Here's how the part is built. I have some questions about the finished solid (model axes, mm). A direction names the side the tool comes from. Round coordinates to 2 decimals unless told otherwise and drop trailing zeros. Order: outer loops, then holes, each group sorted by start corner. A loop starts at its lowest first (then second) coordinate and runs counter-clockwise, first axis right, second up.
```python
from build123d import *

# Parameters (mm, degrees)
F0_W     = 137.8
F0_H     = 2.4
F3_DEPTH = 62.9
F4_START = -61.7
F4_DEPTH = 1.2


with BuildPart() as f1:
    # F0 (on Top) → F1 (revolve)
    with BuildSketch(Plane.XY):
        with Locations((0, 1.2)):
            Rectangle(F0_W, F0_H)
    revolve(axis=Axis((-37.6928597689, 0, 0), (1, 0, 0)))

    # F2 (on Right) → F3 (join, symmetric)
    with BuildSketch(Plane.YZ):
        Polygon((-32.72, -2.4), (0, -2.4), (0, -0.8), (-7, -0.8), (-32.72, -0.8), align=None)
    extrude(amount=F3_DEPTH, both=True)

    # F2 (on Right) → F4 (join)
    with BuildSketch(Plane.YZ.offset(F4_START)):
        Polygon((-7, -0.8), (0, -0.8), (0, 0.1875793553), (-7, 0.8), align=None)
    extrude(amount=-F4_DEPTH)

    # F5: F1 across plane


with BuildPart() as f1_1:
    add(f1.part)
    add(f1.part.mirror(Plane.YZ))


solid = f1_1.part
```
1) I'm going to push flat-ended pins straight in: pin 1 (0.5 mm diameter, centred on y = -5, z = 0, fed in from +X); pin 2 (1.3 mm diameter, centred on x = -62.5, z = 0, fed in from -Y); pin 3 (1.5 mm diameter, centred on y = -17.5, z = 1, fed in from -X); pin 4 (1.5 mm diameter, centred on y = -4, z = -1.5, fed in from -X). Where does each tip first touch, or does it pass through?
2) If we section it at A-A (x = 47.5): Write out the boundary of the cut face in (y, z).
3) For faces 1 (the flat face through (68.9, 0, 0)), 2 (the cylindrical face through (0.965, 1.29, 2.024)), which set-ups out of +Z, -Z, +X, -X, +Y, -Y let a thin tool reach every point of the face, with its end or its side?
4) I need wall thicknesses on line 1 (Z direction, x = -8, y = -15); line 2 (X direction, y = -29, z = -1.25); line 3 (Y direction, x = -50, z = 0). Which ranges of each line are inside material? Lowest first, please.
Solutions:
1. pin 1: stops at x = 62.9
1. pin 2: stops at y = -7
1. pin 3: passes through
1. pin 4: stops at x = -62.9
2. outline: (-32.72, -2.4) - (0, -2.4) arc R2.4 ccw (long way) to (-2.26, -0.8) - (-32.72, -0.8) - close
3. face 1: +Z, -Z, +X, +Y, -Y
3. face 2: none
4. line 1: z = -2.4 to -0.8
4. line 2: x = -62.9 to 62.9
4. line 3: y = -2.4 to 2.4
